Could you check a few things on this model? Use its own coordinates, in mm. Face numbers are marked on the shaded views. Coordinates: 2 decimals unless noted, no trailing zeros. Loops run counter-clockwise (first coordinate to the right, second up) from the corner with the lowest first, then second, coordinate; pieces in that order, holes last. Notation, with made-up numbers: (83, -31) -> (106, -31) arc R22 ccw to (106, -16) -> close; hole circle Ø9 at (81, 1.25). An arc over 180 degrees is marked (long way). One line per question, with ' | ' between items.
from build123d import *

# Parameters (mm, degrees)
SKETCH1_R           = 2.286
BOSS_EXTRUDE1_DEPTH = 95.25
SKETCH2_W           = 82.55
SKETCH2_H           = 9.906
CUT_EXTRUDE1_DEPTH  = 11.922


with BuildPart() as part:
    # Sketch1 → Boss-Extrude1 (new body)
    with BuildSketch(Plane.XY):
        with BuildLine():
            Line((0, 0), (10.922, 0))
            Line((10.922, 0), (10.922, 7.62))
            ThreePointArc((10.922, 7.62), (5.461, 13.081), (0, 7.62))
            Line((0, 7.62), (0, 0))
        make_face()
        with Locations((5.461, 7.62)):
            Circle(SKETCH1_R, mode=Mode.SUBTRACT)
    extrude(amount=BOSS_EXTRUDE1_DEPTH)

    # Sketch2 → Cut-Extrude1 (cut, through all)
    with BuildSketch(Plane(origin=(10.922, 0, 0), x_dir=(0, 0, -1), z_dir=(1, 0, 0))):
        with Locations((-47.625, 8.128)):
            Rectangle(SKETCH2_W, SKETCH2_H)
    extrude(amount=-CUT_EXTRUDE1_DEPTH, mode=Mode.SUBTRACT)


solid = part.part
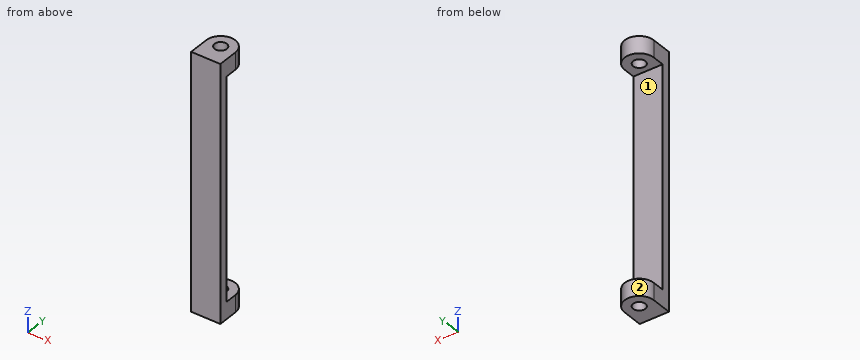
1) If we section it at B-B on x = 8.75: Please give me the cut outline in (y, z) (3 decimals).
Data:
outline: (0, 0) -> (11.979, 0) -> (11.979, 6.35) -> (3.175, 6.35) -> (3.175, 88.9) -> (11.979, 88.9) -> (11.979, 95.25) -> (0, 95.25) -> close
2) We'd pull the mould along Z, two halves only. Please class the marked faces 1 and 2: pulls with the +Z half, pulls with the -Z half, needs draft (parallel to the pull), parting line crosses it, or undercut.
Data:
face 1: undercut | face 2: needs draft
3) If we section it at A-A on y = 12.25: Please give me the cut outline in (x, z).
Data:
outline: (2.57, 0) -> (8.36, 0) -> (8.36, 6.35) -> (2.57, 6.35) -> close; (2.57, 88.9) -> (8.36, 88.9) -> (8.36, 95.25) -> (2.57, 95.25) -> close
4) If we section it at C-C on z = 11: Please give me the cut outline in (x, y) (3 decimals).
Data:
outline: (0, 0) -> (10.922, 0) -> (10.922, 3.175) -> (0, 3.175) -> close
5) I need wall thicknesses on line 1 along Z through (x, y) = (8.75, 6.25); line 2 along Y through (x, z) = (8.25, 76.5) (3 decimals). Which ranges of each line are inside material? Lowest first, please. Write a range as from..to.
Data:
line 1: 0..6.35, 88.9..95.25 | line 2: 0..3.175
